For this review, take the finished solid that the model builds, in its own axes (mm). A direction names the side the tool comes from. Round coordinates to 2 decimals unless told otherwise and drop trailing zeros. Write each loop counter-clockwise with the first axis right and the second up, starting at its lowest first coordinate (ties: lowest second). Pieces come first, ordered by that corner, then holes. Notation, with made-up numbers: (27, 17.25) - (49, 17.25) arc R26 cw to (49, 40.25) - close; hole circle Ø8 at (1.25, 28). An arc over 180 degrees is marked (long way). One line per item, written item: value. Start each with the question number.
Q1. Add section C-C on x = 4.15. Write out the cut boundary in (y, z).
Q2. Mouldability with a two-part tool opening along Y and no side actions: class faces 4 (the face through (2.96, -5.97, -42.27)), 5 (the face through (2.96, -0.96, -43.31)), 6 (the face through (2.96, 11.67, -3.15)) as +Y half, -Y half, draft (parallel to the pull), parting line (faces both ways), or undercut.
Q3. Tool access review of faces 1 (the face through (3, 8, -44)), 2 (the face through (3, -8, -19)), 3 (the face through (3, 2, 4)): name each direction out of +Z, -Z, +X, -X, +Y, -Y from which nothing blocks a thin tool from reaching the whole face with its end or side.
Q4. Add section A-A on z = -41. Write out the cut boundary in (x, y).
Q5. Add section B-B on y = 1.25. Write out the cut boundary in (x, z).
Q6. Add section D-D on y = 12. Write out the cut boundary in (x, z).
Q7. For probe 1 along Z at (x, y) = (4.9, -2); probe 2 along Z at (x, y) = (1, 1.25); probe 3 along X at (y, z) = (0.25, -22), list the stretches that pass through material, from the lowest coordinate up.
Q8. Clearance check with flat-ended pins moving along their axes: pin 1 Ø16 at (y, z) = (9.5, -25.5) entering from +X; pin 2 Ø1.5 at (x, z) = (4, -13.5) entering from +Y; pin 3 Ø1 at (x, y) = (1, -1.5) entering from +Z. State where each tip first meets the part, or that it passes through.
```python
from build123d import *

# Parameters (mm, degrees)
SKETCH1_R           = 3.55
SKETCH1_R_2         = 4
SKETCH1_R_3         = 2.5
SKETCH1_R_4         = 1.5
BOSS_EXTRUDE1_DEPTH = 6
SKETCH2_R           = 4.99
CUT_EXTRUDE1_DEPTH  = 3
SKETCH3_R           = 12.55
CUT_EXTRUDE2_DEPTH  = 3


with BuildPart() as part:
    # Sketch1 → Boss-Extrude1 (new body)
    with BuildSketch(Plane(origin=(0, 0, 0), x_dir=(0, 0, -1), z_dir=(1, 0, 0))):
        with BuildLine():
            Line((-4.410283071, 6.674533934), (10.924994259, 16.807513206))
            ThreePointArc((10.924994259, 16.807513206), (22.222626062, 18.983884909), (31.738603868, 12.517104832))
            ThreePointArc((31.738603868, 12.517104832), (35.34906679, 9.201450356), (40.101489768, 8))
            Line((40.101489768, 8), (47, 8))
            Line((47, 8), (47, -4))
            Line((47, -4), (37.4, -8))
            Line((37.4, -8), (0, -8))
            ThreePointArc((0, -8), (-7.66147086, -2.302577744), (-4.410283071, 6.674533934))
        make_face()
        with Locations((21.931712199, 12)):
            Circle(SKETCH1_R, mode=Mode.SUBTRACT)
        Circle(SKETCH1_R_2, mode=Mode.SUBTRACT)
        with Locations((41, 0)):
            Circle(SKETCH1_R_3, mode=Mode.SUBTRACT)
        with Locations((29.919099476, 9.092828782)):
            Circle(SKETCH1_R_4, mode=Mode.SUBTRACT)
        with Locations((13.944324923, 14.907171218)):
            Circle(SKETCH1_R_4, mode=Mode.SUBTRACT)
    extrude(amount=BOSS_EXTRUDE1_DEPTH)

    # Sketch2 → Cut-Extrude1 (cut)
    with BuildSketch(Plane(origin=(6, 0, 0), x_dir=(0, 0, -1), z_dir=(1, 0, 0))):
        Circle(SKETCH2_R)
    extrude(amount=-CUT_EXTRUDE1_DEPTH, mode=Mode.SUBTRACT)

    # Sketch3 → Cut-Extrude2 (cut)
    with BuildSketch(Plane(origin=(6, 0, 0), x_dir=(0, 0, -1), z_dir=(1, 0, 0))):
        with Locations((21.931712199, 12)):
            Circle(SKETCH3_R)
    extrude(amount=-CUT_EXTRUDE2_DEPTH, mode=Mode.SUBTRACT)


solid = part.part
```
Result set:
1. outline: (-8, -37.4) - (-4, -47) - (8, -47) - (8, -40.1) arc R10 cw to (9.86, -34.3) arc R12.55 cw (long way) to (16.29, -10.14) - (6.67, 4.41) arc R8 ccw to (-8, 0) - close; hole circle Ø9.98 at (0, 0); hole circle Ø5 at (0, -41)
2. face 4: -Y half
2. face 5: undercut
2. face 6: +Y half
3. face 1: -Z, +X, -X, +Y
3. face 2: +Z, -Z, +X, -X, -Y
3. face 3: +X
4. outline: (0, -6.5) - (6, -6.5) - (6, -2.5) - (0, -2.5) - close; (0, 2.5) - (6, 2.5) - (6, 8) - (0, 8) - close
5. outline: (0, -47) - (6, -47) - (6, -43.17) - (0, -43.17) - close; (0, -38.83) - (6, -38.83) - (6, -28.41) - (3, -28.41) - (3, -15.46) - (6, -15.46) - (6, -4.83) - (3, -4.83) - (3, -3.8) - (0, -3.8) - close; (0, 3.8) - (3, 3.8) - (3, 4.83) - (6, 4.83) - (6, 7.9) - (0, 7.9) - close
6. outline: (0, -32.1) - (3, -32.1) - (3, -25.48) - (0, -25.48) - close; (0, -18.38) - (3, -18.38) - (3, -9.38) - (6, -9.38) - (6, -3.65) - (0, -3.65) - close
7. probe 1: z = -47 to -42.5, -39.5 to -4.57, 4.57 to 7.75
7. probe 2: z = -47 to -43.17, -38.83 to -3.8, 3.8 to 7.9
7. probe 3: x = 0 to 3
8. pin 1: stops at x = 3
8. pin 2: stops at y = 3.44
8. pin 3: stops at z = 7.94
